from build123d import *
from build123d.topology import SkipClean

# Parameters (mm, degrees)
SKETCH1_R                 = 1.6500000000000006
SKETCH1_R_2               = 6.25
SKETCH1_R_3               = 1.6500000000000004
BOSS_EXTRUDE1_DEPTH       = 2
BOSS_EXTRUDE2_START       = 2
BOSS_EXTRUDE2_OUTLINE_R   = 7.5
BOSS_EXTRUDE2_OUTLINE_R_2 = 6.25
BOSS_EXTRUDE2_DEPTH       = 38
CUT_EXTRUDE2_START        = 2
SKETCH1_4_R               = 2.8
SKETCH1_4_R_2             = 2.8000000000000003
SKETCH1_4_R_3             = 2.7999999999999994
SKETCH1_4_R_4             = 2.8000000000000016
CUT_EXTRUDE2_DEPTH        = 8
CUT_EXTRUDE3_START        = 2
SKETCH1_5_R               = 2.8
SKETCH1_5_R_2             = 2.7999999999999994
SKETCH1_5_R_3             = 2.8000000000000016
CUT_EXTRUDE3_DEPTH        = 46.314258622305886
FILLET1_R                 = 1.5


# Read off the part's stored shape, not the designer's step: Boss-Extrude2
with BuildPart() as part:
    # Sketch1 → Boss-Extrude1 (new body)
    with BuildSketch(Plane(origin=(0, 0, 0), x_dir=(0, 0, -1), z_dir=(1, 0, 0))):
        with BuildLine():
            ThreePointArc((-9.235679756024062, 7.263932780812693), (-6.819714318196267, 7.1682440093196265), (-5.379034853060263, 5.226469558848167))
            ThreePointArc((-5.37903485305997, 5.226469558848125), (-6.495190528383201, 3.7500000000001563), (-7.215772836598412, 2.0451460511681123))
            ThreePointArc((-7.215772836598439, 2.0451460511681465), (-9.617738571694561, 2.3219238414507375), (-10.908590197578363, 4.366366899528586))
            ThreePointArc((-10.908590197578294, 4.366366899528582), (-10.175798494467182, -5.8749999999999565), (-1.672910441554004, -11.630299680340986))
            ThreePointArc((-1.6729104415540204, -11.630299680341029), (-2.7980242534982347, -9.490167850770279), (-1.836737983538199, -7.271615610016004))
            ThreePointArc((-1.8367379835382087, -7.271615610015976), (-1.38e-15, -7.500000000000001), (1.8367379835382058, -7.271615610015976))
            ThreePointArc((1.8367379835381987, -7.271615610016002), (2.798024253498237, -9.49016785077028), (1.6729104415540168, -11.630299680341032))
            ThreePointArc((1.672910441553996, -11.630299680340986), (10.175798494467136, -5.8750000000000355), (10.908590197578357, 4.366366899528418))
            ThreePointArc((10.908590197578427, 4.3663668995284235), (9.617738571694534, 2.3219238414505634), (7.215772836598344, 2.0451460511680883))
            ThreePointArc((7.2157728365984, 2.0451460511681567), (6.495190528383213, 3.7500000000001346), (5.379034853060037, 5.226469558848057))
            ThreePointArc((5.379034853060338, 5.226469558848102), (6.81971431819637, 7.168244009319535), (9.235679756024162, 7.263932780812571))
            ThreePointArc((9.235679756024219, 7.263932780812644), (7.994e-14, 11.750000000000004), (-9.235679756024119, 7.26393278081277))
        make_face()
        with Locations((-8.127648414516955, -4.692500000000004)):
            Circle(SKETCH1_R, mode=Mode.SUBTRACT)
        Circle(SKETCH1_R_2, mode=Mode.SUBTRACT)
        with Locations((8.127648414516958, -4.692499999999999)):
            Circle(SKETCH1_R, mode=Mode.SUBTRACT)
        with Locations((-1.7e-16, 9.385)):
            Circle(SKETCH1_R_3, mode=Mode.SUBTRACT)
    extrude(amount=BOSS_EXTRUDE1_DEPTH)

    # Boss-Extrude2 outline → Boss-Extrude2 (add)
    with BuildSketch(Plane(origin=(0, 0, 0), x_dir=(0, 0, -1), z_dir=(1, 0, 0)).offset(BOSS_EXTRUDE2_START)):
        Circle(BOSS_EXTRUDE2_OUTLINE_R)
        Circle(BOSS_EXTRUDE2_OUTLINE_R_2, mode=Mode.SUBTRACT)
    extrude(amount=BOSS_EXTRUDE2_DEPTH)

    # Sketch1<4> → Cut-Extrude2 (cut)
    with BuildSketch(Plane(origin=(0, 0, 0), x_dir=(0, 0, -1), z_dir=(1, 0, 0)).offset(CUT_EXTRUDE2_START)):
        with Locations((1.15e-15, -9.385)):
            Circle(SKETCH1_4_R)
        with Locations((-8.127648414517033, -4.692499999999865)):
            Circle(SKETCH1_4_R_2)
        with Locations((-8.127648414516935, 4.692500000000037)):
            Circle(SKETCH1_4_R_3)
        with Locations((6.439e-14, 9.385)):
            Circle(SKETCH1_4_R)
        with Locations((8.127648414517003, 4.692499999999925)):
            Circle(SKETCH1_4_R_4)
        with Locations((8.127648414516901, -4.692500000000093)):
            Circle(SKETCH1_4_R_3)
    extrude(amount=CUT_EXTRUDE2_DEPTH, mode=Mode.SUBTRACT)

    # Sketch1<5> → Cut-Extrude3 (cut, through all)
    with SkipClean():  # the faces are left unmerged after this step: merging them gives an invalid solid
        with BuildSketch(Plane(origin=(0, 0, 0), x_dir=(0, 0, -1), z_dir=(1, 0, 0)).offset(CUT_EXTRUDE3_START)):
            with Locations((1.15e-15, -9.385)):
                Circle(SKETCH1_5_R)
            with Locations((-8.127648414516935, 4.692500000000037)):
                Circle(SKETCH1_5_R_2)
            with Locations((8.127648414517003, 4.692499999999925)):
                Circle(SKETCH1_5_R_3)
        extrude(amount=-CUT_EXTRUDE3_DEPTH, mode=Mode.SUBTRACT)

    # Fillet1
    # the kernel refuses this fillet: 1.5 mm, written as the material it takes off along each edge
    with BuildSketch(Plane(origin=(40, 0, 0), x_dir=(0, 0, -1), z_dir=(0, -1, 0))) as fillet1_piece_1:
        with BuildLine():
            CenterArc((7.75, -1.4790199457750504), FILLET1_R, 99.59406822685953, 80.40593177314048)
            Line((7.500000000000024, -1.4211e-13), (7.495000000000024, 0.02958039891535691))
            ThreePointArc((7.495000000000024, 0.02958039891535691), (6.875000000000012, 0.03000000000000114), (6.25, 0.03000000000000114))
            Line((6.25, 0.03000000000000114), (6.22, 0))
            Line((6.22, 0), (6.22, -1.4790199457750504))
            Line((6.22, -1.4790199457750504), (6.25, -1.4790199457750504))
        make_face()
    revolve(axis=Axis((40, 0, 0), (1, 0, 0)), mode=Mode.SUBTRACT)


solid = part.part
Check sheet for the modelled part. Datum: model origin and axes. Units: mm. A direction names the side the tool comes from. Coordinates: 2 decimals unless noted, no trailing zeros. Write each loop counter-clockwise with the first axis right and the second up, starting at its lowest first coordinate (ties: lowest second). Pieces come first, ordered by that corner, then holes.
Item 1: Scan lines: probe 1 along Y at (x, z) = (1.45, 0) (3 decimals); probe 2 along Z at (x, y) = (23.5, -0.25) (3 decimals); probe 3 along X at (y, z) = (-1.5, -7.5). Record each from-to range of solid material in increasing order.
Numbers:
probe 1: y = -6.585 to -6.25, 6.25 to 7.735, 11.035 to 11.75
probe 2: z = -7.496 to -6.245, 6.245 to 7.496
probe 3: x = 0 to 2
Item 2: Cross-section at C-C on y = 0. Record the boundary of the cut face in (x, z).
Numbers:
outline: (0, -11.75) - (2, -11.75) - (2, -7.5) - (40, -7.5) arc R1.5 ccw to (38.52, -6.25) - (0, -6.25) - close; (0, 6.25) - (38.52, 6.25) arc R1.5 ccw to (40, 7.5) - (2, 7.5) - (2, 11.75) - (0, 11.75) - close
Item 3: Cross-section at A-A on z = 0. Record the boundary of the cut face in (x, y) (3 decimals).
Numbers:
outline: (0, -6.585) - (10, -6.585) - (10, -7.5) - (40, -7.5) arc R1.5 ccw to (38.521, -6.25) - (0, -6.25) - close; (0, 6.25) - (38.521, 6.25) arc R1.5 ccw to (40, 7.5) - (10, 7.5) - (10, 6.585) - (2, 6.585) - (2, 7.735) - (0, 7.735) - close; (0, 11.035) - (2, 11.035) - (2, 11.75) - (0, 11.75) - close
Item 4: Cross-section at D-D on z = -8.25. Record the boundary of the cut face in (x, y).
Numbers:
outline: (0, -8.37) - (2, -8.37) - (2, -6.34) - (0, -6.34) - close; (0, -3.05) - (2, -3.05) - (2, 1.9) - (0, 1.9) - close; (0, 7.49) - (2, 7.49) - (2, 8.37) - (0, 8.37) - close
Item 5: Depth check by flat-ended pin: pin 1 Ø0.6 at (y, z) = (3.5, -6) entering from -X; pin 2 Ø4 at (x, z) = (10.5, 3.5) entering from +Y; pin 3 Ø2 at (x, y) = (34.5, -2.5) entering from +Z; pin 4 Ø2.5 at (y, z) = (-4.69, -8.13) entering from +X. Enter the tip coordinate at first touch or a pass-through.
Numbers:
pin 1: stops at x = 10
pin 2: stops at y = 7.35
pin 3: stops at z = 7.35
pin 4: passes through
Item 6: Mould release check, pull along Z, two halves, no side actions. Record for faces 4 (the face through (0.986, -6.003, -10.101)), 5 (the face through (25, 5.1, 5.5)), 6 (the face through (5.944, 6.585, 0.028)), 7 (the face through (0, -5, 5)): released by +Z, released by -Z, zero draft, split by the parting line, or undercut.
Numbers:
face 4: released by -Z
face 5: split by the parting line
face 6: undercut
face 7: zero draft
Item 7: Access from +Z, -Z, +X, -X, +Y, -Y to the whole of each face (thin tool, end or side, straight path). Record for faces 1 (the face through (5.9, -3.3, 5.7)), 2 (the face through (10, 7, 0)), 3 (the face through (5.9, -3.3, -5.7)).
Numbers:
face 1: +Z
face 2: +Y
face 3: -Z
